Verification items for the finished model (mm, model axes). Face numbers are marked on the shaded views. A direction names the side the tool comes from. Coordinates: 2 decimals unless noted, no trailing zeros. Loops run counter-clockwise (first coordinate to the right, second up) from the corner with the lowest first, then second, coordinate; pieces in that order, holes last. Notation, with made-up numbers: (33, -9.75) - (81, -9.75) arc R7 cw to (81, -0.75) - close; hole circle Ø6 at (46, 61). An arc over 180 degrees is marked (long way). Answer as CSV lines item,"result". Start each with the question number.
1. Gauge pin test, flat ends, axial feed: P1, Ø6, axis at y = 16.5, z = -14, coming from the +X side; P2, Ø3, axis at y = 21, z = -6.5, coming from the +X side; P3, Ø1.2, axis at x = 10, y = 1, coming from the -Z side; P4, Ø5, axis at x = 9, z = 8.5, coming from the -Y side. Record the tip position at first contact, or that the pin passes through.
2. Set-up check for the marked faces 1 and 2: record each of +Z, -Z, +X, -X, +Y, -Y from which the full face is reachable in a straight line by a thin tool's end or side.
3. Cross-section at C-C (x = -34.5). Enter the section's corners in (y, z).
4. Material ranges on line 1 (X direction, y = 1.5, z = 5.25) (3 decimals); line 2 (Y direction, x = 21.5, z = -14.5); line 3 (Z direction, x = -18.75, y = 1.8) (3 decimals), recorded low to high. Write a range as [from, to].
5. Cross-section at B-B (y = -2.5). Enter the section's corners in (x, z), plus the area to 3 significant figures.
6. Release check for a two-part mould opening along Y. For the marked faces 3, 4 and 5 record: pulls with the +Y half, pulls with the -Y half, needs draft (parallel to the pull), parting line crosses it, or undercut.
7. Cross-section at A-A (x = -18.75). Enter the section's corners in (y, z) (1 decimal).
8. Cross-section at D-D (z = -16). Enter the section's corners in (x, y), plus the area to 3 significant figures.
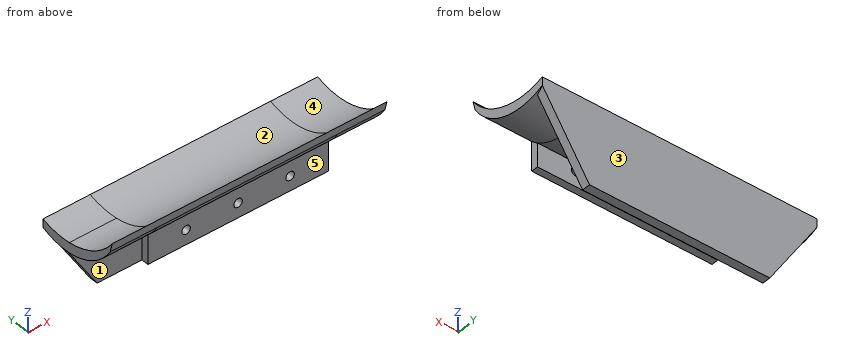
Autodesk Inventor part; units mm, degrees
ref_plane "YZ Plane" through (0, 0, 0) normal (1, 0, 0) x (0, 1, 0)
ref_plane "XZ Plane" through (0, 0, 0) normal (0, 1, 0) x (-1, 0, 0)
ref_plane "XY Plane" through (0, 0, 0) normal (0, 0, 1) x (1, 0, 0)
sketch "Sketch1" plane through (0, 0, 0) normal (0, 1, 0) x (-1, 0, 0)
  line L0 (0, 0) -> (32.5, 0)
  line L1 (32.5, 0) -> (-32.5, 0)
  line L2 (-32.5, 0) -> (-32.5, 19)
  line L3 (-32.5, 19) -> (32.5, 19)
  line L4 (32.5, 19) -> (32.5, 0)
  dimension "d0" = 32.5
  dimension "d1" = 65
  dimension "d2" = 19
extrude "Extrusion1" add sketch "Sketch1" along normal blind 25
sketch "Sketch2" plane through (32.5, 0, 19) normal (1, 0, 0) x (0, 0, -1)
  line L0 (19, 0) -> (8, 0)
  line L1 (0, 0) -> (19, 0)
  line L2 (8, 0) -> (0, -2.143594)
  line L3 (0, -2.143594) -> (0, 0)
  dimension "d5" = 11
  dimension "d6" = 165
extrude "Extrusion2" add sketch "Sketch2" against normal up to surface (65 mm away)
sketch "Sketch3" plane through (32.5, 0, 0) normal (1, 0, 0) x (0, 0, -1)
  line L0 (-19, -2.143594) -> (-19, 25)
  line L1 (-19, 25) -> (0, 25)
  line L2 (-19, 25) -> (-19, -5)
  arc A0 (-19, -5) -> (-9.5, 25) centre (-33.73129, 16.169075) ccw
  line L3 (-19, -2.143594) -> (-11, 0)
  line L4 (-19, -5) -> (-11, 0)
  line L5 (-19, -2.143594) -> (-19, 25)
  line L6 (-19, 25) -> (-9.5, 25)
  point P0 (0, 0)
  point P1 (-14.409764, -0.913643)
  dimension "d59" = 30
extrude "Extrusion3" cut sketch "Sketch3" against normal blind 81.4375 contours L0 L1 A0 L3
sketch "Sketch4" plane through (0, 0, 0) normal (0, -1, 0) x (1, 0, 0)
  line L0 (-32.5, 0) -> (-32.5, 11)
  line L1 (-32.5, 0) -> (-32.5, 10.5)
  line L2 (-32.5, 10.5) -> (32.5, 10.5)
  line L3 (32.5, 11) -> (32.5, 0)
  line L4 (-32.5, 0) -> (-32.5, 5.25)
  line L5 (-32.5, 5.25) -> (32.5, 5.25)
  line L6 (-32.5, 5.25) -> (-18.75, 5.25)
  line L7 (-18.75, 5.25) -> (0, 5.25)
  line L8 (0, 5.25) -> (18.75, 5.25)
  line L9 (18.75, 5.25) -> (32.5, 5.25)
  circle A0 centre (18.75, 5.25) radius 1.525
  circle A1 centre (0, 5.25) radius 1.525
  circle A2 centre (-18.75, 5.25) radius 1.525
  point P0 (0, 0)
  point P1 (-17.225, 5.25)
  point P2 (-20.275, 5.25)
  point P3 (1.525, 5.25)
  point P4 (-1.525, 5.25)
  point P5 (20.275, 5.25)
  point P6 (17.225, 5.25)
  dimension "d12" = 10.5
  dimension "d13" = 5.25
  dimension "d14" = 13.75
  dimension "d15" = 18.75
  dimension "d16" = 18.75
  dimension "d17" = 3.05
  dimension "d18" = 3.05
  dimension "d19" = 3.05
extrude "Extrusion4" cut sketch "Sketch4" against normal blind 4 contours A2 L5 | L5 A2 | A1 L5 | L5 A1 | A0 L5 | L5 A0
sketch "Sketch5" plane through (32.5, 0, 0) normal (0, 0, -1) x (-1, 0, 0)
  line L0 (0, 25) -> (65, 25)
  line L1 (65, 25) -> (65, -2.143594)
  line L2 (0, 25) -> (65, 25)
  line L3 (65, 25) -> (65, 22)
  line L4 (65, 22) -> (0, 22)
  line L5 (0, 22) -> (0, 25)
  point P0 (32.5, 0)
  dimension "d22" = 3
sketch "Sketch6" plane through (32.5, 0, 0) normal (1, 0, 0) x (0, 0, -1)
  line L0 (0, 0) -> (-11, 0)
  line L1 (0, 0) -> (-10, 0)
  line L2 (-11, 0) -> (0, 0)
  line L3 (-19, 25) -> (0, 25)
  arc A0 (-11, 0) -> (-6.906688, 25) centre (-24.791662, 15.093247) ccw
  line L4 (0, 0) -> (0, 25)
  line L5 (0, 25) -> (0, 22)
  line L6 (0, 22) -> (-5.548149, 22)
  line L7 (0, 0) -> (0, 2.5)
  line L8 (0, 2.5) -> (-8.68495, 2.5)
  point P0 (-9.5, 25)
  dimension "d23" = 10
  dimension "d24" = 3
  dimension "d25" = 2.5
extrude "Extrusion5" cut sketch "Sketch6" against normal blind 113.5375 contours L8 A0 L6 L4
extrude "Extrusion6" add sketch "Sketch5" along normal blind 20
sketch "Sketch12" plane through (0, 25, 0) normal (0, 1, 0) x (1, 0, 0)
  line L0 (0, 0) -> (0, -9.5)
  line L1 (49.5, -9.5) -> (-49.5, -9.5)
  line L2 (0, -9.5) -> (0, 0)
  line L3 (0, -9.5) -> (0, -6)
  line L4 (0, -6) -> (8.228384, -6)
  line L5 (8.228384, -6) -> (-5.400421, -6)
  dimension "d85" = 3.5
sketch "Sketch14" plane through (32.5, 0, 11) normal (1, 0, 0) x (0, 0, -1)
  line L0 (11, 0) -> (0, 0)
  line L1 (0, 0) -> (9.434, 0) construction
  arc A0 (-3.409764, -0.913643) -> (1.5, 25) centre (-22.73129, 16.169075) ccw
  line L2 (1.5, 25) -> (31, 25)
  arc A1 (-8.000486, -4.999258) -> (1.5, 25) centre (-22.726506, 16.168322) ccw
  line L3 (-3.409764, -0.913643) -> (0, 0)
  line L4 (-3.409764, -0.913643) -> (0, 0)
  line L5 (-8.000486, -4.999258) -> (-4.590768, -4.085627)
  line L6 (-8.000486, -4.999258) -> (-4.470486, -4.999258) construction
  line L7 (-4.590768, -4.085627) -> (0, 0)
  point P0 (28, 25)
  point P1 (-2.386043, 0.31942)
  dimension "d60" = 9.434
  dimension "d62" = 3.53
  dimension "d63" = 15
extrude "Extrusion12" add sketch "Sketch14" against normal up to surface (65 mm away)
sketch "Sketch15" plane through (32.5, 0, 0) normal (1, 0, 0) x (0, 0, -1)
  arc A0 (-19.000486, -4.999258) -> (-13.386043, 0.31942) centre (-33.726506, 16.168322) ccw
  line L0 (-9.5, 25) -> (20, 25)
  arc A1 (-19.000486, -4.999258) -> (-9.5, 25) centre (-33.729569, 16.169292) ccw
  line L1 (-9.5, 25) -> (-6.5, 25)
  line L2 (-19.000486, -4.999258) -> (-15.590768, -4.085627)
  arc A2 (-15.590768, -4.085627) -> (-6.5, 25) centre (-27.017687, 15.44936) ccw
  line L3 (-15.590768, -4.085627) -> (-11, 0)
  line L4 (-19.000486, -4.999258) -> (-15.590768, -4.085627)
  line L5 (-9.5, 25) -> (-6.5, 25)
  line L6 (-9.5, 25) -> (20, 25)
  point P0 (0, 0)
  point P1 (17, 25)
  dimension "d66" = 3
extrude "Extrusion13" add sketch "Sketch15" against normal blind 65
sketch "Sketch16" plane through (32.5, 0, 0) normal (1, 0, 0) x (0, 0, -1)
  line L0 (-19.000486, -4.999258) -> (-15.590768, -4.085627)
  arc A0 (-8.067422, 13.618284) -> (-9.5, 25) centre (-33.73129, 16.169075) ccw
  arc A1 (-19.000486, -4.999258) -> (-9.5, 25) centre (-33.729569, 16.169292) ccw
  line L1 (-9.5, 25) -> (20, 25)
  line L2 (-9.5, 25) -> (-6.5, 25)
  arc A2 (-15.590768, -4.085627) -> (-10.479625, 0) centre (-27.017687, 15.44936) ccw
  arc A3 (-6.108674, 6.78891) -> (-4.450402, 17.154601) centre (-24.791662, 15.093247) ccw
  arc A4 (-15.590768, -4.085627) -> (-6.5, 25) centre (-27.017687, 15.44936) ccw
  line L3 (-19.000486, -4.999258) -> (-15.590768, -4.085627)
  line L4 (-9.5, 25) -> (-6.5, 25)
  point P0 (0, 0)
  point P1 (17, 25)
  point P2 (-10.479625, 0)
  dimension "d69" = 3
sketch "Sketch16 outline for Extrusion14" plane through (32.5, 0, 0) normal (1, 0, 0) x (0, 0, -1)
  arc A0 (-10.479625, 0) -> (-6.5, 25) centre (-27.017687, 15.44936) ccw
  arc A1 (-15.590768, -4.085627) -> (-10.479625, 0) centre (-27.017687, 15.44936) ccw
  line L0 (-19.000486, -4.999258) -> (-15.590768, -4.085627)
  arc A2 (-9.5, 25) -> (-19.000486, -4.999258) centre (-33.729569, 16.169292) cw
  line L1 (-6.5, 25) -> (-9.5, 25)
extrude "Extrusion14" add sketch "Sketch16 outline for Extrusion14" along normal blind 17
sketch "Sketch17" plane through (-32.5, 0, 0) normal (-1, 0, 0) x (0, 0, 1)
  line L0 (9.5, 25) -> (-20, 25)
  line L1 (19.000486, -4.999258) -> (15.590768, -4.085627)
  arc A0 (8.067422, 13.618284) -> (19.000486, -4.999258) centre (33.729569, 16.169292) ccw
  arc A1 (9.5, 25) -> (19.000486, -4.999258) centre (33.729569, 16.169292) ccw
  line L2 (9.5, 25) -> (6.5, 25)
  arc A2 (4.450402, 17.154601) -> (6.108674, 6.78891) centre (24.791662, 15.093247) ccw
  arc A3 (6.5, 25) -> (15.590768, -4.085627) centre (27.017687, 15.44936) ccw
  line L3 (15.590768, -4.085627) -> (19.000486, -4.999258)
  point P0 (0, 0)
  point P1 (-17, 25)
  dimension "d72" = 3
sketch "Sketch17 outline for Extrusion15" plane through (-32.5, 0, 0) normal (-1, 0, 0) x (0, 0, 1)
  arc A0 (6.5, 25) -> (15.590768, -4.085627) centre (27.017687, 15.44936) ccw
  line L0 (9.5, 25) -> (6.5, 25)
  arc A1 (8.067422, 13.618284) -> (9.5, 25) centre (33.729569, 16.169292) cw
  arc A2 (19.000486, -4.999258) -> (8.067422, 13.618284) centre (33.729569, 16.169292) cw
  line L1 (15.590768, -4.085627) -> (19.000486, -4.999258)
extrude "Extrusion15" add sketch "Sketch17 outline for Extrusion15" along normal blind 17
sketch "Sketch18" plane through (-32.5, 15.093247, 24.791662) normal (-1, 0, 0) x (0, 0.1579684, 0.9874442)
  arc A0 (-16.497042, 12.67187) -> (-18.101737, 9.890438) centre (2.25433, 0) ccw
  arc A1 (-18.11904, -9.854746) -> (-16.516593, -12.64289) centre (2.25433, 0) ccw
  arc A2 (-18.101737, 9.890438) -> (-18.11904, -9.854746) centre (2.25433, 0) ccw
  arc A3 (-19.76023, 5.248748) -> (-19.76023, -5.248748) centre (2.25433, 0) ccw
  arc A4 (-19.76023, 5.248748) -> (-19.76023, -5.248748) centre (0, 0) ccw
  point P0 (-26.864638, -10.98744)
sketch "Sketch18 outline for Extrusion16" plane through (-32.5, 15.093247, 24.791662) normal (-1, 0, 0) x (0, 0.1579684, 0.9874442)
  arc A0 (-19.76023, 5.248748) -> (-19.76023, -5.248748) centre (0, 0) ccw
  arc A1 (-19.76023, -5.248748) -> (-19.76023, 5.248748) centre (2.25433, 0) cw
extrude "Extrusion16" cut sketch "Sketch18 outline for Extrusion16" against normal blind 66.2125
sketch "Sketch20" plane through (0, 25, 0) normal (0, 1, 0) x (1, 0, 0)
  arc A0 (32.5, 17) -> (29.5, 20) centre (29.5, 17) ccw
  line L0 (32.5, -6.5) -> (49.5, -6.5)
  line L1 (-32.5, 20) -> (-32.5, -5.354831)
  line L2 (49.5, -6.5) -> (32.5, -6.5)
  line L3 (-32.5, -6.5) -> (-32.5, -5.354831)
  line L4 (-32.5, 17) -> (-32.5, -6.5)
  line L5 (-32.5, -6.5) -> (-49.5, -6.5)
  line L6 (32.5, -6.5) -> (32.5, 20)
  line L7 (32.5, 17) -> (32.5, -6.5)
  line L8 (32.5, 20) -> (49.5, -6.5)
  line L9 (-32.5, 20) -> (32.5, 20)
  line L10 (-32.5, 20) -> (-49.5, -6.5)
  point P0 (0, 0)
sketch "Sketch21" plane through (-49.5, 0, 0) normal (-1, 0, 0) x (0, 0, 1)
  arc A0 (9.5, 25) -> (19.000486, -4.999258) centre (33.729569, 16.169292) ccw
  line L0 (9.5, 25) -> (19.000486, -4.999258)
  point P0 (0, 0)
extrude "Extrusion18" cut sketch "Sketch21" against normal blind 124.3
extrude "Extrusion19" add sketch "Sketch20" against normal up to surface (3 mm away) contours L6 L8 L0 | L1 L3 L5 L10
properties part number "slope"
Values follow:
1,P1,"passes through"
1,P2,"stops at x = 41.88"
1,P3,"stops at z = 0"
1,P4,"stops at y = -0.54"
2,face 1,"-Z, +X, -X"
2,face 2,"+Z, +X, -X"
3,outline,"(-5, 19) - (-4.09, 15.59) arc R22.63 ccw to (22, 5.35) - (22, -16.88) - (25, -16.88) - (25, 9.5) arc R25.79 cw to (13.62, 8.07) arc R25.79 cw to start"
4,line 1,"x = [-32.5, -20.275], [-17.225, -1.525], [1.525, 17.225], [20.275, 32.5]"
4,line 2,"y = [22, 25]"
4,line 3,"z = [0, 3.725], [6.775, 12.315]"
5,outline,"(-49.5, 13.23) - (49.5, 13.23) - (49.5, 15.94) - (32.5, 15.94) - (-49.5, 15.94) - close"
5,area,"268 mm²"
6,face 3,"pulls with the +Y half"
6,face 4,"undercut"
6,face 5,"pulls with the -Y half"
7,outline,"(-5, 19) - (-4.1, 15.6) arc R22.6 ccw to (0, 10.5) - (0, 6.8) - (2.5, 6.8) - (2.5, 8.5) arc R22.6 ccw to (22, 5.4) - (22, -20) - (25, -20) - (25, 9.5) arc R25.8 cw to (-0.9, 14.4) arc R25.8 cw to start; (0, 0) - (2.5, 0) - (2.5, 3.7) - (0, 3.7) - close"
8,outline,"(-35.07, 22) - (35.07, 22) - (35.07, 25) - (-35.07, 25) - close"
8,area,"210 mm²"
